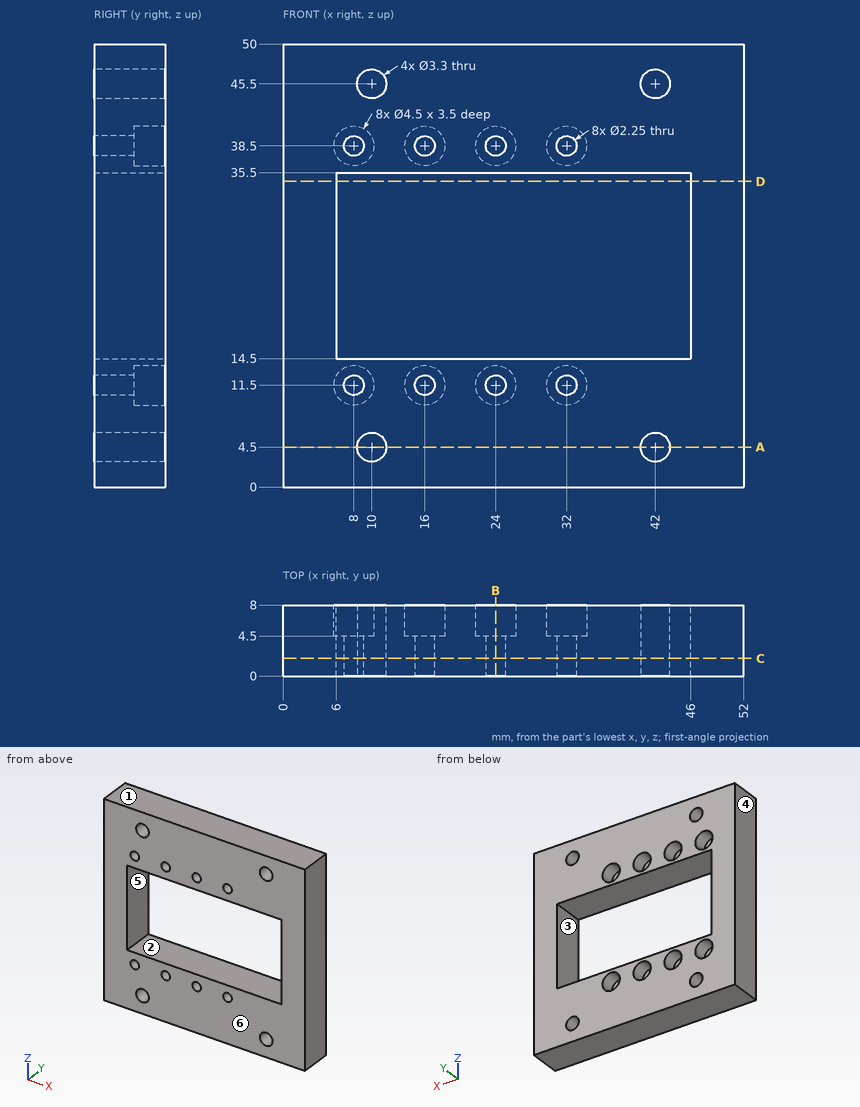
Here's the drawing with two shaded views (mm, measured from the low corner). I have some questions. A direction names the side the tool comes from. Coordinates: 2 decimals unless noted, no trailing zeros. Write each loop counter-clockwise with the first axis right and the second up, starting at its lowest first coordinate (ties: lowest second). Pieces come first, ordered by that corner, then holes. Notation, with made-up numbers: (-6, -18) -> (49, -18) arc R32 cw to (49, 14) -> close; hole circle Ø4 at (49.25, 10.5). An arc over 180 degrees is marked (long way). Use a Markdown table: item, result. Add a question column.
(1) If we section it at C-C, the plane y = 2: State how many separate pieces and enclosed holes the cut face has, and give its area (3 significant figures).
(2) Please list where these lines run through material, in increasing order: line 1 (Z direction, x = 8, y = 1.55) (3 decimals); line 2 (X direction, y = 3.6, z = 38.5) (3 decimals); line 3 (Z direction, x = 10, y = 3.75).
(3) If we section it at A-A, the plane z = 4.5: Write out the boundary of the cut face in (x, y), and give its area (3 significant figures).
(4) We'd pull the mould along Z, two halves only. Please class the marked faces 1, 2, 3 and 4: +Z half, -Z half, draft (parallel to the pull), parting line (faces both ways), or undercut.
(5) I'm going to push a flat-ended pin straight in: P1, Ø1.3, axis at x = 23, z = 12, coming from the +Y side. Where does the tip first touch, or does it pass through?
(6) For the marked faces 5 and 6, which set-ups out of +Z, -Z, +X, -X, +Y, -Y let a thin tool reach every point of the face, with its end or its side?
(7) If we section it at B-B, the plane x = 24: Write out the boundary of the cut face in (y, z) (3 decimals).
(8) If we section it at D-D, the plane z = 34.5: Write out the boundary of the cut face in (x, y), and give its area (3 significant figures).
Outcome:
| question | item | result |
|---|---|---|
| 1 | separate pieces | 1 |
| 1 | enclosed holes | 13 |
| 1 | area | 1,690 mm^2 |
| 2 | line 1 | z = 0 to 10.375, 12.625 to 14.5, 35.5 to 37.375, 39.625 to 50 |
| 2 | line 2 | x = 0 to 6.875, 9.125 to 14.875, 17.125 to 22.875, 25.125 to 30.875, 33.125 to 52 |
| 2 | line 3 | z = 0 to 2.85, 6.15 to 14.5, 35.5 to 43.85, 47.15 to 50 |
| 3 | outline | (0, 0) -> (8.35, 0) -> (8.35, 8) -> (0, 8) -> close; (11.65, 0) -> (40.35, 0) -> (40.35, 8) -> (11.65, 8) -> close; (43.65, 0) -> (52, 0) -> (52, 8) -> (43.65, 8) -> close |
| 3 | area | 363 mm^2 |
| 4 | face 1 | +Z half |
| 4 | face 2 | undercut |
| 4 | face 3 | undercut |
| 4 | face 4 | draft |
| 5 | P1 | stops at y = 4.5 |
| 6 | face 5 | +Y, -Y |
| 6 | face 6 | +Z, -Z, +X, -X, -Y |
| 7 | outline | (0, 0) -> (8, 0) -> (8, 9.25) -> (4.5, 9.25) -> (4.5, 10.375) -> (0, 10.375) -> close; (0, 12.625) -> (4.5, 12.625) -> (4.5, 13.75) -> (8, 13.75) -> (8, 14.5) -> (0, 14.5) -> close; (0, 35.5) -> (8, 35.5) -> (8, 36.25) -> (4.5, 36.25) -> (4.5, 37.375) -> (0, 37.375) -> close; (0, 39.625) -> (4.5, 39.625) -> (4.5, 40.75) -> (8, 40.75) -> (8, 50) -> (0, 50) -> close |
| 8 | outline | (0, 0) -> (6, 0) -> (6, 8) -> (0, 8) -> close; (46, 0) -> (52, 0) -> (52, 8) -> (46, 8) -> close |
| 8 | area | 96.0 mm^2 |
